```python
from build123d import *

# Parameters (mm, degrees)
SKETCH1_W           = 93
SKETCH1_H           = 81
BOSS_EXTRUDE1_DEPTH = 24
SKETCH2_R           = 1.6
CUT_EXTRUDE1_DEPTH  = 24
SKETCH3_W           = 17
SKETCH3_H           = 10
CUT_EXTRUDE2_DEPTH  = 20


with BuildPart() as part:
    # Sketch1 → Boss-Extrude1 (new body)
    with BuildSketch(Plane(origin=(0, 0, 0), x_dir=(1, 0, 0), z_dir=(0, 1, 0))):
        Rectangle(SKETCH1_W, SKETCH1_H)
    extrude(amount=BOSS_EXTRUDE1_DEPTH)

    # Sketch2 → Cut-Extrude1 (cut)
    with BuildSketch(Plane(origin=(0, 24, 0), x_dir=(1, 0, 0), z_dir=(0, 1, 0))):
        with Locations(Location((-41.5, 38.5, 0), (0, 0, 270))):
            Circle(SKETCH2_R)
        with Locations(Location((-41.5, -38.5, 0), (0, 0, 90))):
            Circle(SKETCH2_R)
        with Locations(Location((41.5, -38.5, 0), (0, 0, 270))):
            Circle(SKETCH2_R)
        with Locations(Location((41.5, 38.5, 0), (0, 0, 90))):
            Circle(SKETCH2_R)
    extrude(amount=-CUT_EXTRUDE1_DEPTH, mode=Mode.SUBTRACT)

    # Sketch3 → Cut-Extrude2 (cut)
    with BuildSketch(Plane(origin=(46.5, 0, 0), x_dir=(0, 0, -1), z_dir=(1, 0, 0))):
        with Locations((-10, 16)):
            Rectangle(SKETCH3_W, SKETCH3_H)
    extrude(amount=-CUT_EXTRUDE2_DEPTH, mode=Mode.SUBTRACT)


solid = part.part
```
For this review, take the finished solid that the model builds, in its own axes (mm). A direction names the side the tool comes from. Coordinates: 2 decimals unless noted, no trailing zeros. Loops run counter-clockwise (first coordinate to the right, second up) from the corner with the lowest first, then second, coordinate; pieces in that order, holes last. Notation, with made-up numbers: (-14.5, 52) - (1.5, 52) arc R23 cw to (1.5, 71) - close; hole circle Ø6 at (72, 20). An arc over 180 degrees is marked (long way). Use one line per item in the form item = value. Start each with the question number.
1) Take a section at B-B (y = 14). State the section outline as (x, z) points, plus the area to 3 significant figures.
2) To check wall thickness, follow probe 1 along X at (y, z) = (8.25, 38.5); probe 2 along X at (y, z) = (12.25, 9.5). State the ranges of each line that lie inside material, in increasing order. Write a range as from..to.
3) Take a section at A-A (x = 41.5). State the section outline as (y, z) points.
4) For faces 1 (the face through (37, 21, 10)), 2 (the face through (-46.5, 12, 1)), list the 3-axis set-ups (+Z, -Z, +X, -X, +Y, -Y) from which the entire face can be reached by the end or side of a thin tool; tool diameter is ignored.
5) For pin 1 (18.5 mm diameter, centred on x = 36, z = 10, fed in from -Y); pin 2 (1.9 mm diameter, centred on x = 41.5, z = 38.5, fed in from -Y); pin 3 (1 mm diameter, centred on y = 13.5, z = 11, fed in from +X), all flat-tipped, find the tip position at first contact; note any pin that passes through.
6) Draft analysis for pull direction Y (two halves, no side actions). For faces 3 (the face through (-1, 24, -1)), 4 (the face through (37, 16, 1.5)), 5 (the face through (-1, 0, -1)), 6 (the face through (-42.92, 12.17, -37.76)), state which applies: released by +Y, released by -Y, zero draft, split by the parting line, or undercut.
7) Take a section at D-D (x = -41.5). State the section outline as (y, z) points.
8) Take a section at C-C (z = 38.5). State the section outline as (x, y) points.
From the geometry:
q1.outline = (-46.5, -40.5) - (46.5, -40.5) - (46.5, 1.5) - (26.5, 1.5) - (26.5, 18.5) - (46.5, 18.5) - (46.5, 40.5) - (-46.5, 40.5) - close; hole circle Ø3.2 at (-41.5, -38.5); hole circle Ø3.2 at (-41.5, 38.5); hole circle Ø3.2 at (41.5, -38.5); hole circle Ø3.2 at (41.5, 38.5)
q1.area = 7,160 mm2
q2.probe_1 = -46.5..-43.1, -39.9..39.9, 43.1..46.5
q2.probe_2 = -46.5..26.5
q3.outline = (0, -40.5) - (24, -40.5) - (24, -40.1) - (0, -40.1) - close; (0, -36.9) - (24, -36.9) - (24, 36.9) - (0, 36.9) - close; (0, 40.1) - (24, 40.1) - (24, 40.5) - (0, 40.5) - close; hole (11, 1.5) - (21, 1.5) - (21, 18.5) - (11, 18.5) - close
q4.face_1 = +X
q4.face_2 = +Z, -Z, -X, +Y, -Y
q5.pin_1 = 0
q5.pin_2 = through
q5.pin_3 = 26.5
q6.face_3 = released by +Y
q6.face_4 = undercut
q6.face_5 = released by -Y
q6.face_6 = zero draft
q7.outline = (0, -40.5) - (24, -40.5) - (24, -40.1) - (0, -40.1) - close; (0, -36.9) - (24, -36.9) - (24, 36.9) - (0, 36.9) - close; (0, 40.1) - (24, 40.1) - (24, 40.5) - (0, 40.5) - close
q8.outline = (-46.5, 0) - (-43.1, 0) - (-43.1, 24) - (-46.5, 24) - close; (-39.9, 0) - (39.9, 0) - (39.9, 24) - (-39.9, 24) - close; (43.1, 0) - (46.5, 0) - (46.5, 24) - (43.1, 24) - close
